```python
from build123d import *

# Parameters (mm, degrees)
SKETCH1_R           = 1.6
BOSS_EXTRUDE1_DEPTH = 0.8
CUT_EXTRUDE1_DEPTH  = 0.8


with BuildPart() as part:
    # Sketch1 → Boss-Extrude1 (new body)
    with BuildSketch(Plane.XY):
        Polygon((-21.328326925, 35.64702685), (-59.328326925, 35.64702685), (-59.328326925, 29.04702685), (-67.028326925, 29.04702685), (-67.028326925, -9.15297315), (-62.528326925, -9.15297315), (-62.528326925, -15.15297315), (-67.028326925, -15.15297315), (-67.028326925, -53.25297315), (-59.428326925, -53.25297315), (-59.428326925, -60.85297315), (-21.428326925, -60.85297315), (-21.428326925, -56.35297315), (-15.428326925, -56.35297315), (-15.428326925, -60.85297315), (22.571673075, -60.85297315), (22.571673075, -53.25297315), (29.471673075, -53.25297315), (29.471673075, -15.073036827), (24.971673075, -15.073036827), (24.971673075, -9.073036827), (29.471673075, -9.073036827), (29.471673075, 28.94702685), (22.671673075, 28.94702685), (22.671673075, 35.64702685), (-15.328326925, 35.64702685), (-15.328326925, 31.14702685), (-21.328326925, 31.14702685), align=None)
        with Locations((-18.428147066, -47.449600232)):
            Circle(SKETCH1_R, mode=Mode.SUBTRACT)
        with Locations((-53.624954006, -12.252793292)):
            Circle(SKETCH1_R, mode=Mode.SUBTRACT)
        with Locations((-5.370945752, 1.09702685)):
            Circle(SKETCH1_R, mode=Mode.SUBTRACT)
        with Locations((16.768659873, -12.252793292)):
            Circle(SKETCH1_R, mode=Mode.SUBTRACT)
        with Locations((-18.428147066, 22.944013647)):
            Circle(SKETCH1_R, mode=Mode.SUBTRACT)
    extrude(amount=BOSS_EXTRUDE1_DEPTH)

    # Sketch2 → Cut-Extrude1 (cut)
    with BuildSketch(Plane.XY.offset(0.8)):
        Polygon((-7.935255139, -9.545182739), (-16.420536513, -1.059901365), (-18.130934836, -2.770299688), (-9.645653462, -11.255581062), align=None)
        Polygon((-5.036117336, -6.646044936), (-13.52139871, 1.839236438), (-16.420536513, -1.059901365), (-7.935255139, -9.545182739), align=None)
        Polygon((-3.35240311, -4.96233071), (-11.837684484, 3.522950664), (-13.52139871, 1.839236438), (-5.036117336, -6.646044936), align=None)
    extrude(amount=-CUT_EXTRUDE1_DEPTH, mode=Mode.SUBTRACT)


solid = part.part
```
Design review of the part built by this model. Coordinates are the model's own, in mm. A direction names the side the tool comes from. Round coordinates to 2 decimals unless told otherwise and drop trailing zeros. Put each result on its own line as item: value.
Q1. Draft analysis for pull direction X (two halves, no side actions). For faces 3 (the face through (-19, -12, 0)), 4 (the face through (-14.94, 0.42, 0.41)), state which applies: released by +X, released by -X, zero draft, split by the parting line, or undercut.
Reported:
face 3: zero draft
face 4: undercut
Q2. Consider section A-A (z = 0.3). State how many separate pieces and enclosed holes the cut face has, and give its area (3 significant figures).
Reported:
separate pieces: 1
enclosed holes: 6
area: 8,850 mm²
Q3. Machinability: for faces 1 (the face through (-6.54, -8.15, 0.41)), 2 (the face through (-19, -12, 0.8)), which of the approach directions +Z, -Z, +X, -X, +Y, -Y give a long, thin tool a straight path to every point of the face, cutting with its end or side? Answer none if there is none.
Reported:
face 1: +Z, -Z
face 2: +Z, +X, -X, +Y, -Y
Q4. Insertion check: pin 1 Ø1.9 at (x, y) = (16.77, -12.25) entering from -Z; pin 2 Ø3 at (x, y) = (-30.5, -46) entering from -Z. Each pin has a flat end and moves straight along its axis. Give the tip position at first contact, or say it passes through.
Reported:
pin 1: through
pin 2: z = 0
Q5. To check wall thickness, follow line 1 (Y direction, x = -63, z = 0.1); line 2 (X direction, y = 1.5, z = 0.3); line 3 (X direction, y = 22.5, z = 0.75). State the ranges of each line that lie inside material, in increasing order.
Reported:
line 1: -53.25 to -15.15, -9.15 to 29.05
line 2: -67.03 to -13.86, -9.81 to -6.92, -3.82 to 29.47
line 3: -67.03 to -19.97, -16.89 to 29.47
